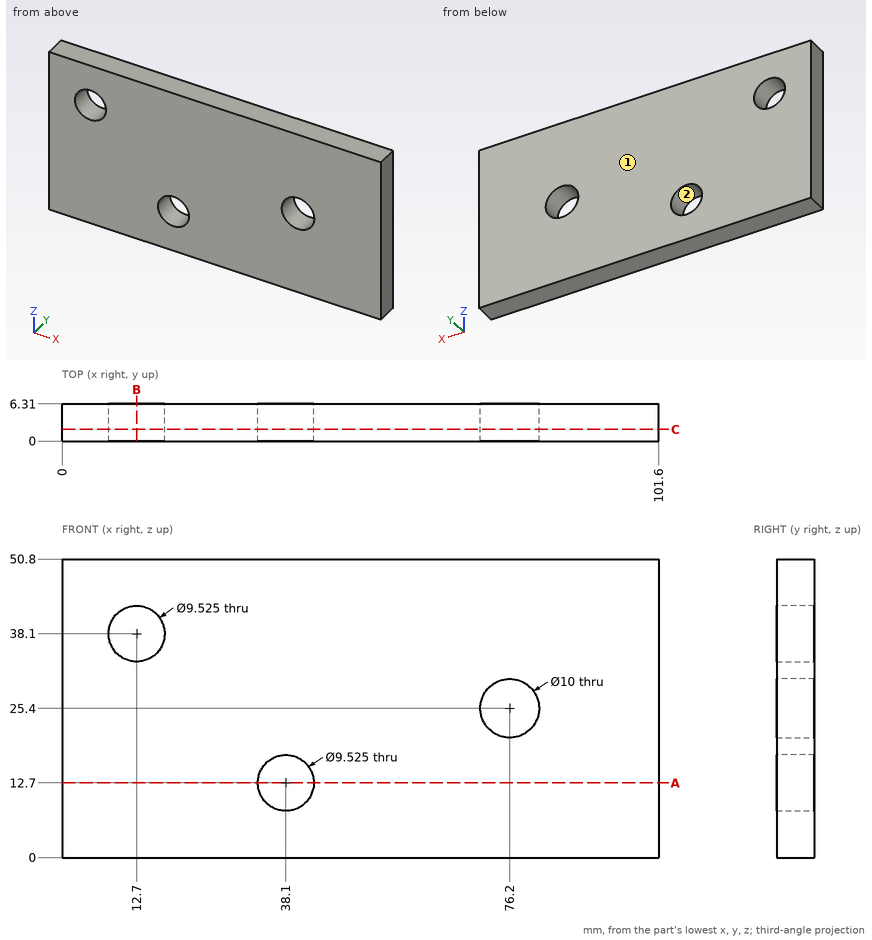
Geometry check sheet. Reference: drawing and pictorial views, mm from the part's lowest x, y, z. Round coordinates to 2 decimals unless told otherwise and drop trailing zeros. Order: outer loops, then holes, each group sorted by start corner. A loop starts at its lowest first (then second) coordinate and runs counter-clockwise, first axis right, second up. Notation, with made-up numbers: (-24.5, 79.25) - (10.5, 79.25) arc R16 ccw to (10.5, 93.25) - close; hole circle Ø2 at (-28.75, 66.25). An arc over 180 degrees is marked (long way). Use a Markdown table: item, result. Add a question column.
1) Section check B-B (x = 12.7). Record the cut outline in (y, z).
2) Section check A-A (z = 12.7). Record the cut outline in (x, y).
3) Gauge pin test, flat end, axial feed: P1, Ø9, axis at x = 76.2, z = 25.4, coming from the +Y side. Record the tip position at first contact, or that the pin passes through.
4) Mould release check, pull along X, two halves, no side actions. Record for the marked faces 1 and 2: released by +X, released by -X, zero draft, split by the parting line, or undercut.
5) Thickness scan on line 1 along X through (y, z) = (3.5, 38.1); line 2 along X through (y, z) = (3, 12.7); line 3 along Z through (x, y) = (76.2, 4). Record the ranges inside material, lowest first.
6) Section check C-C (y = 2). Record the cut outline in (x, z) (1 decimal), then the cut area to 3 significant figures.
Established:
| question | item | result |
|---|---|---|
| 1 | outline | (0, 0) - (6.31, 0) - (6.31, 33.34) - (0, 33.34) - close; (0, 42.86) - (6.31, 42.86) - (6.31, 50.8) - (0, 50.8) - close |
| 2 | outline | (0, 0) - (33.34, 0) - (33.34, 6.31) - (0, 6.31) - close; (42.86, 0) - (101.6, 0) - (101.6, 6.31) - (42.86, 6.31) - close |
| 3 | P1 | through |
| 4 | face 1 | zero draft |
| 4 | face 2 | undercut |
| 5 | line 1 | 0 to 7.94, 17.46 to 101.6 |
| 5 | line 2 | 0 to 33.34, 42.86 to 101.6 |
| 5 | line 3 | 0 to 20.4, 30.4 to 50.8 |
| 6 | outline | (0, 0) - (101.6, 0) - (101.6, 50.8) - (0, 50.8) - close; hole circle Ø9.5 at (12.7, 38.1); hole circle Ø9.5 at (38.1, 12.7); hole circle Ø10 at (76.2, 25.4) |
| 6 | area | 4,940 mm2 |
